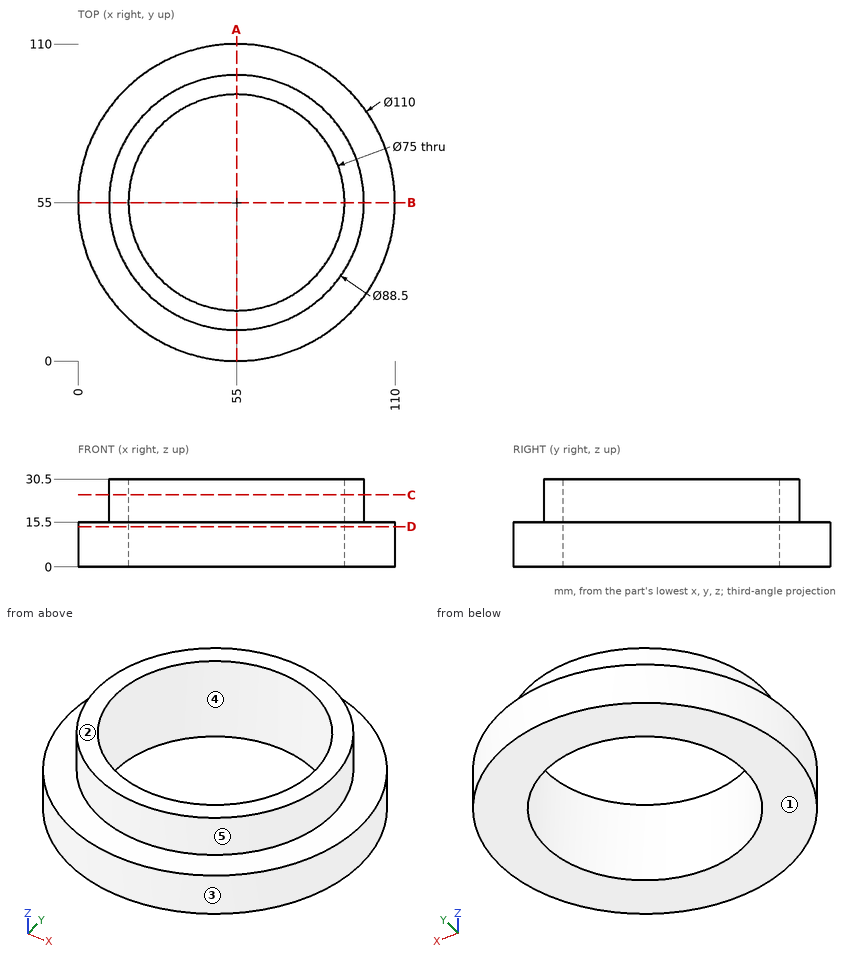
Could you check a few things on this drawing? It's one solid part, dimensions in mm from its lowest x, y, z. A direction names the side the tool comes from. Round coordinates to 2 decimals unless told otherwise and drop trailing zeros. Write each loop counter-clockwise with the first axis right and the second up, starting at its lowest first coordinate (ties: lowest second). Pieces come first, ordered by that corner, then holes.
Q1. Which directions (+Z, -Z, +X, -X, +Y, -Y) give clear straight access to the entire face, cutting with the end or side of a thin tool? Please do the marked faces 4 and 5.
Q2. Will these pins go through, and if not, where does the flat tip stop? P1, Ø1, axis at x = 68.5, z = 22, coming from the +Y side; P2, Ø2, axis at x = 65.5, z = 22.5, coming from the -Y side; P3, Ø1, axis at x = 68.5, z = 7.5, coming from the -Y side.
Q3. If we section it at D-D on z = 14: Write out the boundary of the cut face in (x, y), plus the area to 3 significant figures.
Q4. If we section it at A-A on x = 55: Write out the boundary of the cut face in (y, z), plus the area to 3 significant figures.
Q5. If we mould it in two halves opening along Z, with no side actions, what happens to the marked faces 1, 2 and 3? For each: +Z half, -Z half, draft (parallel to the pull), parting line (faces both ways), or undercut.
Q6. Please list where these lines run through material, in increasing order: probe 1 along Y at (x, z) = (55, 17); probe 2 along Y at (x, z) = (55, 12); probe 3 along X at (y, z) = (28.5, 29.5).
Q7. If we section it at C-C on z = 25: Write out the boundary of the cut face in (x, y), plus the area to 3 significant figures.
Answer below:
1. face 4: +Z, -Z
1. face 5: +Z
2. P1: stops at y = 97.3
2. P2: stops at y = 11.78
2. P3: stops at y = 1.56
3. outline: circle Ø110 at (55, 55); hole circle Ø75 at (55, 55)
3. area: 5,090 mm2
4. outline: (0, 0) - (17.5, 0) - (17.5, 30.5) - (10.75, 30.5) - (10.75, 15.5) - (0, 15.5) - close; (92.5, 0) - (110, 0) - (110, 15.5) - (99.25, 15.5) - (99.25, 30.5) - (92.5, 30.5) - close
4. area: 745 mm2
5. face 1: -Z half
5. face 2: +Z half
5. face 3: draft
6. probe 1: y = 10.75 to 17.5, 92.5 to 99.25
6. probe 2: y = 0 to 17.5, 92.5 to 110
6. probe 3: x = 19.56 to 28.47, 81.53 to 90.44
7. outline: circle Ø88.5 at (55, 55); hole circle Ø75 at (55, 55)
7. area: 1,730 mm2
